```python
from build123d import *

# Parameters (mm, degrees)
F1_DEPTH = 18
F2_R     = 5.25
F3_DEPTH = 25


with BuildPart() as f1:
    # F0 (on Front) → F1 (new body, symmetric)
    with BuildSketch(Plane.XZ):
        with BuildLine():
            ThreePointArc((-18.027756, 6), (0, 19), (18.027756, 6))
            Line((18.027756, 6), (21.027756, 6))
            Line((21.027756, 6), (21.027756, 18))
            Line((21.027756, 18), (43, 18))
            Line((43, 18), (43, 28))
            Line((43, 28), (22.627417, 28))
            ThreePointArc((22.627417, 28), (0, 36), (-22.627417, 28))
            Line((-22.627417, 28), (-43, 28))
            Line((-43, 28), (-43, 18))
            Line((-43, 18), (-21.027756, 18))
            Line((-21.027756, 18), (-21.027756, 6))
            Line((-21.027756, 6), (-18.027756, 6))
        make_face()
    extrude(amount=F1_DEPTH, both=True)

    # F2 (on face) → F3 (cut)
    with BuildSketch(Plane.XY.offset(28)):
        with Locations((-31, 0)):
            Circle(F2_R)
        with Locations((31, 0)):
            Circle(F2_R)
    extrude(amount=-F3_DEPTH, mode=Mode.SUBTRACT)

    # F4 (on Front) → F5 (revolve, cut)
    with BuildSketch(Plane.XZ):
        Polygon((3, 40.073246), (0, 40.122432), (0, 17.161723), (1.5, 17.161723), (1.5, 24.356959), (3, 25.856959), align=None)
    revolve(axis=Axis((0, 0, 25.428471), (0, 0, -1)), mode=Mode.SUBTRACT)


solid = f1.part
```
The listing builds one solid part. Answer for the finished solid, in the listing's coordinates (mm). A direction names the side the tool comes from. Coordinates: 2 decimals unless noted, no trailing zeros. Loops run counter-clockwise (first coordinate to the right, second up) from the corner with the lowest first, then second, coordinate; pieces in that order, holes last. Notation, with made-up numbers: M 70,-28 L 124,-28 A27 ccw 124,3 Z; hole C 17,61.25 d5. An arc over 180 degrees is marked long. Answer as a JSON object with one key per item and string values. Group by question number.
Item 1: Section B-B (z = 15.5) is taken. Write down the section's boundary in (x, y), and give its area (3 significant figures).
Item 2: Section D-D (z = 21.5) is taken. Write down the section's boundary in (x, y), and give its area (3 significant figures).
Item 3: Which of the six approach directions +Z, -Z, +X, -X, +Y, -Y give full straight-line access (tool end or side, diameter ignored) to faces 1 (the face through (-1.5, -0.07, 21.69)), 2 (the face through (-35, -4, 18)), 3 (the face through (-3, 0, 31)), 4 (the face through (21.028, 0, 12)), 5 (the face through (37, 0, 28))?
Item 4: Each of these flat-tipped pins is pushed along its axis until it touches: P1, Ø5.5, axis at x = 0, y = 0, coming from the -Z side; P2, Ø2.5, axis at x = 0, y = 0, coming from the +Z side; P3, Ø1.5, axis at y = 10, z = 13, coming from the -X side; P4, Ø6.5, axis at x = -35.5, y = 1.5, coming from the -Z side. Where does it stop, or does it pass through?
Item 5: Determine the mould class of faces 6 (the face through (25.755, 0.231, 23.07)), 7 (the face through (-1, 18, 25)), 8 (the face through (-21.028, 0, 12)) for opening direction X: +X half, -X half, draft (parallel to the pull), parting line (faces both ways), or undercut.
Item 6: Section A-A (x = -31) is taken. Write down the section's boundary in (y, z).
Item 7: Section C-C (y = 0) is taken. Write down the section's boundary in (x, z), and give its area (3 significant figures).
Item 8: Consider L1, parallel to Y at x = 31, z = 22.5; L2, parallel to Y at x = 0, z = 21; L3, parallel to Z at x = -25, y = -13. Determine where each line is inside the solid, lowest interval first.
Solved:
{
 "1": {"outline": "M -21.03,-18 L -10.99,-18 L -10.99,18 L -21.03,18 Z; M 10.99,-18 L 21.03,-18 L 21.03,18 L 10.99,18 Z", "area": "723 mm2"},
 "2": {"outline": "M -43,-18 L 43,-18 L 43,18 L -43,18 Z; hole C -31,0 d10.5; hole C 0,0 d3; hole C 31,0 d10.5", "area": "2,920 mm2"},
 "3": {"face 1": "+Z, -Z", "face 2": "-Z, -X, +Y, -Y", "face 3": "+Z", "face 4": "-Z, +X, +Y, -Y", "face 5": "+Z, +X, +Y, -Y"},
 "4": {"P1": "stops at z = 18.8", "P2": "passes through", "P3": "stops at x = -21.03", "P4": "stops at z = 18"},
 "5": {"face 6": "undercut", "face 7": "draft", "face 8": "-X half"},
 "6": {"outline": "M -18,18 L -5.25,18 L -5.25,28 L -18,28 Z; M 5.25,18 L 18,18 L 18,28 L 5.25,28 Z"},
 "7": {"outline": "M -43,18 L -36.25,18 L -36.25,28 L -43,28 Z; M -25.75,18 L -21.03,18 L -21.03,6 L -18.03,6 A19 cw -1.5,18.94 L -1.5,24.36 L -3,25.86 L -3,35.87 A36 ccw -22.63,28 L -25.75,28 Z; M 1.5,18.94 A19 cw 18.03,6 L 21.03,6 L 21.03,18 L 25.75,18 L 25.75,28 L 22.63,28 A36 ccw 3,35.87 L 3,25.86 L 1.5,24.36 Z; M 36.25,18 L 43,18 L 43,28 L 36.25,28 Z", "area": "976 mm2"},
 "8": {"L1": "y = -18 to -5.25, 5.25 to 18", "L2": "y = -18 to -1.5, 1.5 to 18", "L3": "z = 18 to 28"}
}
